from build123d import *

# Parameters (mm, degrees)
SKETCH1_W               = 80
SKETCH1_H               = 80
BOSS_EXTRUDE1_DEPTH     = 3.175
CUT_EXTRUDE2_DEPTH      = 57.657573413
CUT_EXTRUDE2_DEPTH_BACK = 57.657573413
SKETCH3_W               = 5.333333333
SKETCH3_H               = 3.175
SKETCH3_W_2             = 3.175
SKETCH3_H_2             = 4.91
SKETCH3_W_3             = 5.333333334
SKETCH4_W               = 80.351781832
SKETCH4_H               = 52.368780003
CUT_EXTRUDE3_DEPTH      = 57.657573413


with BuildPart() as part:
    # Sketch1 → Boss-Extrude1 (new body)
    with BuildSketch(Plane.XY):
        Rectangle(SKETCH1_W, SKETCH1_H)
    extrude(amount=BOSS_EXTRUDE1_DEPTH)

    # Sketch3 → Cut-Extrude2 (cut, two sides: drawn at the far end of the back side and taken through both)
    with BuildSketch(Plane.XY.offset(3.175).offset(-CUT_EXTRUDE2_DEPTH_BACK)):
        with Locations((-37.333333334, -38.4125)):
            Rectangle(SKETCH3_W, SKETCH3_H)
        with Locations((-26.666666666, -38.4125)):
            Rectangle(SKETCH3_W, SKETCH3_H)
        with Locations((-38.4125, -29.46)):
            Rectangle(SKETCH3_W_2, SKETCH3_H_2)
        with Locations((-16, -38.4125)):
            Rectangle(SKETCH3_W_3, SKETCH3_H)
        with Locations((-38.4125, -19.64)):
            Rectangle(SKETCH3_W_2, SKETCH3_H_2)
        with Locations((-5.333333334, -38.4125)):
            Rectangle(SKETCH3_W, SKETCH3_H)
        with Locations((-38.4125, -9.82)):
            Rectangle(SKETCH3_W_2, SKETCH3_H_2)
        with Locations((5.333333334, -38.4125)):
            Rectangle(SKETCH3_W, SKETCH3_H)
        with Locations((-38.4125, 0)):
            Rectangle(SKETCH3_W_2, SKETCH3_H_2)
        with Locations((16, -38.4125)):
            Rectangle(SKETCH3_W_3, SKETCH3_H)
        with Locations((-38.4125, 9.82)):
            Rectangle(SKETCH3_W_2, SKETCH3_H_2)
        with Locations((26.666666666, -38.4125)):
            Rectangle(SKETCH3_W, SKETCH3_H)
        with Locations((-38.4125, 19.64)):
            Rectangle(SKETCH3_W_2, SKETCH3_H_2)
        with Locations((37.333333334, -38.4125)):
            Rectangle(SKETCH3_W, SKETCH3_H)
        with Locations((-38.4125, 29.46)):
            Rectangle(SKETCH3_W_2, SKETCH3_H_2)
        with Locations((-37.333333334, 38.4125)):
            Rectangle(SKETCH3_W, SKETCH3_H)
        with Locations((38.4125, -29.46)):
            Rectangle(SKETCH3_W_2, SKETCH3_H_2)
        with Locations((38.4125, -19.64)):
            Rectangle(SKETCH3_W_2, SKETCH3_H_2)
        with Locations((-26.666666666, 38.4125)):
            Rectangle(SKETCH3_W, SKETCH3_H)
        with Locations((38.4125, -9.82)):
            Rectangle(SKETCH3_W_2, SKETCH3_H_2)
        with Locations((-16, 38.4125)):
            Rectangle(SKETCH3_W_3, SKETCH3_H)
        with Locations((38.4125, 0)):
            Rectangle(SKETCH3_W_2, SKETCH3_H_2)
        with Locations((-5.333333334, 38.4125)):
            Rectangle(SKETCH3_W, SKETCH3_H)
        with Locations((38.4125, 9.82)):
            Rectangle(SKETCH3_W_2, SKETCH3_H_2)
        with Locations((5.333333334, 38.4125)):
            Rectangle(SKETCH3_W, SKETCH3_H)
        with Locations((38.4125, 19.64)):
            Rectangle(SKETCH3_W_2, SKETCH3_H_2)
        with Locations((16, 38.4125)):
            Rectangle(SKETCH3_W_3, SKETCH3_H)
        with Locations((38.4125, 29.46)):
            Rectangle(SKETCH3_W_2, SKETCH3_H_2)
        with Locations((26.666666666, 38.4125)):
            Rectangle(SKETCH3_W, SKETCH3_H)
        with Locations((37.333333334, 38.4125)):
            Rectangle(SKETCH3_W, SKETCH3_H)
    extrude(amount=CUT_EXTRUDE2_DEPTH + CUT_EXTRUDE2_DEPTH_BACK, mode=Mode.SUBTRACT)

    # Sketch4 → Cut-Extrude3 (cut, through all)
    with BuildSketch(Plane.XY.offset(3.175)):
        with Locations((0.175890916, -13.909390002)):
            Rectangle(SKETCH4_W, SKETCH4_H)
    extrude(amount=-CUT_EXTRUDE3_DEPTH, mode=Mode.SUBTRACT)


solid = part.part
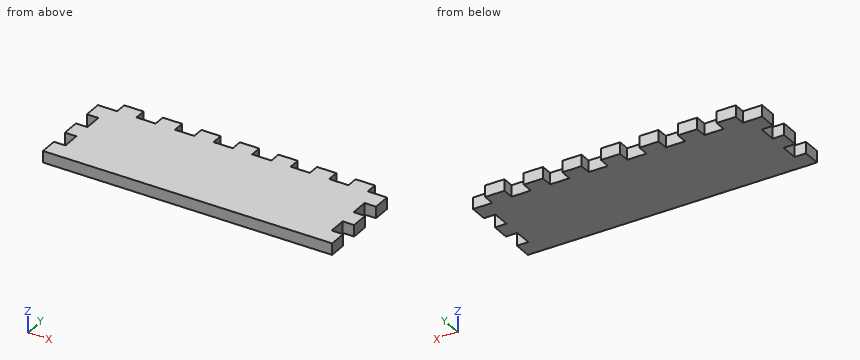
Check sheet for the modelled part. Datum: model origin and axes. Units: mm. Round coordinates to 2 decimals unless told otherwise and drop trailing zeros. Order: outer loops, then holes, each group sorted by start corner. A loop starts at its lowest first (then second) coordinate and runs counter-clockwise, first axis right, second up.
(1) Cross-section at A-A, the plane x = -25. Enter the section's corners in (y, z) (3 decimals), and give its area (3 significant figures).
(2) Scan lines: probe 1 along Y at (x, z) = (26.5, 1) (3 decimals); probe 2 along X at (y, z) = (21.5, 0.4) (3 decimals). Record each from-to range of solid material in increasing order.
(3) Cross-section at B-B, the plane y = 28.75. Enter the section's corners in (x, z) (3 decimals).
(4) Go/stop test with flat-tipped pins: P1, Ø1.6, axis at y = 39, z = 1.5, coming from the -X side; P2, Ø1.6, axis at x = -38.5, z = 2.5, coming from the +Y side (3 decimals); P3, Ø1, axis at y = 30.5, z = 2, coming from the -X side (3 decimals). Record where each tip stops, or that it passes through.
Check sheet entries:
1. outline: (12.275, 0) - (36.825, 0) - (36.825, 3.175) - (12.275, 3.175) - close
1. area: 77.9 mm2
2. probe 1: y = 12.275 to 36.825
2. probe 2: x = -36.825 to 36.825
3. outline: (-36.825, 0) - (36.825, 0) - (36.825, 3.175) - (-36.825, 3.175) - close
4. P1: stops at x = -34.67
4. P2: stops at y = 36.825
4. P3: stops at x = -36.825
